Read the model definition and answer for the solid it produces. Units are mm, in the model's axes. A direction names the side the tool comes from. Round coordinates to 2 decimals unless told otherwise and drop trailing zeros. Write each loop counter-clockwise with the first axis right and the second up, starting at its lowest first coordinate (ties: lowest second). Pieces come first, ordered by that corner, then holes.
Autodesk Inventor part; units mm, degrees
ref_plane "YZ Plane" through (0, 0, 0) normal (1, 0, 0) x (0, 1, 0)
ref_plane "XZ Plane" through (0, 0, 0) normal (0, 1, 0) x (-1, 0, 0)
ref_plane "XY Plane" through (0, 0, 0) normal (0, 0, 1) x (1, 0, 0)
sketch "Sketch1" plane through (0, 0, 0) normal (0, 1, 0) x (-1, 0, 0)
  line L0 (0, 0) -> (80, 0)
  line L1 (80, 0) -> (80, -150)
  line L2 (80, -150) -> (0, -150)
  line L3 (0, -150) -> (0, 0)
  line L4 (0, 0) -> (-5, 0)
  line L5 (-5, 0) -> (-5, -150)
  line L6 (-5, -150) -> (0, -150)
  line L7 (0, -150) -> (0, 0)
  line L8 (0, -6.8284) -> (2.8284, -4)
  circle A0 centre (14, -14) radius 10
  line L9 (2.8284, -4) -> (0, -4)
  line L10 (0, -6.8284) -> (-5, -6.8284)
  line L11 (0, -4) -> (-5, -4)
  dimension "d0" = 150
  dimension "d1" = 80
  dimension "d2" = 5
  dimension "d3" = 4
  dimension "d4" = 45
  dimension "d5" = 20
  dimension "d6" = 4
  dimension "d7" = 14
  dimension "d8" = 14
extrude "Extrusion1" add sketch "Sketch1" along normal blind 4 contours L0 L1 L2 L3 L8 L9 | L9 L8 L3
extrude "Extrusion2" cut sketch "Sketch1" along normal blind 4 contours L9 L8 L3
extrude "Extrusion3" add sketch "Sketch1" along normal blind 2 contours L3 L11 L5 L4 | L3 L10 L5 L11 | L3 L6 L5 L10
extrude "Extrusion4" cut sketch "Sketch1" along normal blind 2 contours L3 L10 L5 L11
properties part number "backWall"
Q1. Straight lines are drawn through the part: probe 1 along Z at (x, y) = (-14, 3.2); probe 2 along X at (y, z) = (2.15, -10.5); probe 3 along Z at (x, y) = (-19, 1.5). For each, find the intervals that lie inside material, in ascending order.
Verdict:
probe 1: z = -150 to -24, -4 to 0
probe 2: x = -80 to -23.37, -4.63 to 0
probe 3: z = -150 to -22.66, -5.34 to 0
Q2. Section B-B (x = -14) is taken. Determine the outline of the cut face in (y, z).
Verdict:
outline: (0, -150) - (4, -150) - (4, -24) - (0, -24) - close; (0, -4) - (4, -4) - (4, 0) - (0, 0) - close
Q3. Flat-ended cylindrical pins translate along their axes: pin 1 Ø2 at (x, y) = (-21, 3.5) entering from +Z; pin 2 Ø2 at (y, z) = (3.5, -1.5) entering from +X; pin 3 Ø2 at (x, z) = (3.5, -1) entering from +Y. Find the tip coordinate at first contact, or state that the pin passes through.
Verdict:
pin 1: stops at z = 0
pin 2: stops at x = 0
pin 3: stops at y = 2
Q4. Determine the mould class of faces 3 (the flat face through (3, 2, -2)), 4 (the flat face through (-1.394, 1.972, -5.434)), 5 (the flat face through (-37, 2, 0)), 6 (the flat face through (-38, 2, -150)) for opening direction Z: pulls with the +Z half, pulls with the -Z half, needs draft (parallel to the pull), parting line crosses it, or undercut.
Verdict:
face 3: needs draft
face 4: undercut
face 5: pulls with the +Z half
face 6: pulls with the -Z half
Q5. Which of the six approach directions +Z, -Z, +X, -X, +Y, -Y give full straight-line access (tool end or side, diameter ignored) to faces 1 (the flat face through (-80, 2, -74)), 2 (the flat face through (3, 2, -77))?
Verdict:
face 1: +Z, -Z, -X, +Y, -Y
face 2: +Z, -Z, +X, +Y
Q6. Section A-A (y = 3.4) is taken. Determine the outline of the cut face in (x, z).
Verdict:
outline: (-80, -150) - (0, -150) - (0, -6.83) - (-2.83, -4) - (0, -4) - (0, 0) - (-80, 0) - close; hole circle Ø20 at (-14, -14)
Q7. Section C-C (z = -14) is taken. Determine the outline of the cut face in (x, y).
Verdict:
outline: (-80, 0) - (-24, 0) - (-24, 4) - (-80, 4) - close; (-4, 0) - (5, 0) - (5, 2) - (0, 2) - (0, 4) - (-4, 4) - close
Q8. Section D-D (z = -75) is taken. Determine the outline of the cut face in (x, y).
Verdict:
outline: (-80, 0) - (5, 0) - (5, 2) - (0, 2) - (0, 4) - (-80, 4) - close
